Source: three-view drawing plus pictorial views. Frame: mm from the lowest corner of the part. A direction names the side the tool comes from. Coordinates: 2 decimals unless noted, no trailing zeros. Write each loop counter-clockwise with the first axis right and the second up, starting at its lowest first coordinate (ties: lowest second). Pieces come first, ordered by that corner, then holes. Notation, with made-up numbers: (-38, 1.5) - (-30, 1.5) arc R16 ccw to (-30, 22.5) - close; hole circle Ø9 at (26, 36). An arc over 180 degrees is marked (long way). Answer as a JSON object with one key per item and string values. Group by question number.
Item 1: Section C-C on y = 0.95. Return loops of the section in (x, z) (1 decimal), and give its area (3 significant figures).
Item 2: Section A-A on x = 3.5. Return loops of the section in (y, z).
Item 3: Section B-B on z = 5.35. Return loops of the section in (x, y).
Item 4: First-contact query: pin 1 Ø2 at (x, y) = (1, 1.5) entering from -Z; pin 2 Ø1 at (x, y) = (3, 1.5) entering from +Z; pin 3 Ø1 at (x, y) = (1, 4.5) entering from +Z. Flat tips, straight axial feed; report the tip coordinate or a pass-through.
Item 5: Mould query, pull axis Y, two halves, no side actions, for the marked faces 1, 2 and 3. Classes: pulls with the +Y half, pulls with the -Y half, needs draft (parallel to the pull), parting line crosses it, or undercut.
Item 6: Line query: line 1 along Y through (x, z) = (0.75, 1.25); line 2 along X through (y, z) = (1.05, 3); line 3 along Y through (x, z) = (1.8, 5.2). Output: solid intervals per line, ascending. Write a range as from..to.
Item 7: Set-up query: the marked faces 4 and 5. Return all of +Z, -Z, +X, -X, +Y, -Y with unobstructed straight access to the full face (end or side cutting, diameter ignored); none if empty.
Item 8: Section D-D on x = 0.5. Return loops of the section in (y, z).
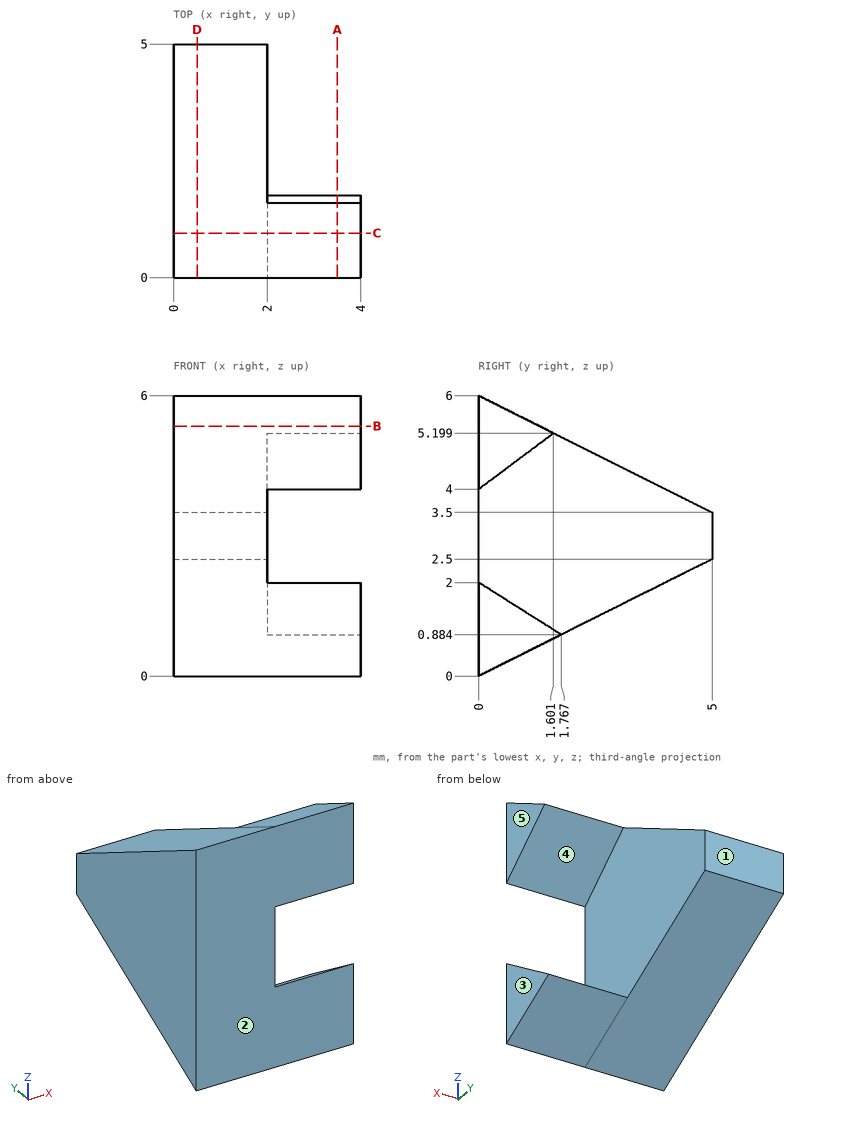
Checks:
{
 "1": {"outline": "(0, 0.5) - (4, 0.5) - (4, 1.4) - (2, 1.4) - (2, 4.7) - (4, 4.7) - (4, 5.5) - (0, 5.5) - close", "area": "13.6 mm^2"},
 "2": {"outline": "(0, 0) - (1.77, 0.88) - (0, 2) - close; (0, 4) - (1.6, 5.2) - (0, 6) - close"},
 "3": {"outline": "(0, 0) - (4, 0) - (4, 1.3) - (0, 1.3) - close"},
 "4": {"pin 1": "z = 0.25", "pin 2": "z = 5.5", "pin 3": "z = 4"},
 "5": {"face 1": "pulls with the +Y half", "face 2": "pulls with the -Y half", "face 3": "needs draft"},
 "6": {"line 1": "0..2.5", "line 2": "0..2", "line 3": "0..1.6"},
 "7": {"face 4": "+X, +Y", "face 5": "+Z, -Z, +X, +Y, -Y"},
 "8": {"outline": "(0, 0) - (5, 2.5) - (5, 3.5) - (0, 6) - close"}
}
